from build123d import *

# Parameters (mm, degrees)
F0_W     = 10
F0_H     = 7.475247
F1_DEPTH = 33.528


with BuildPart() as f1:
    # F0 (on Top) → F1 (new body)
    with BuildSketch(Plane.XY):
        with Locations((-52.5, -26.262377)):
            Rectangle(F0_W, F0_H)
        with Locations((52.5, -26.262377)):
            Rectangle(F0_W, F0_H)
        with BuildLine():
            Line((47.5, 30), (-47.5, 30))
            Line((-47.5, 30), (-47.5, -22.524753))
            Line((-47.5, -22.524753), (-47.5, -30))
            Line((-47.5, -30), (-22.5, -30))
            Line((-22.5, -30), (-22.5, 0))
            Line((-22.5, 0), (-22.5, 16.022185))
            ThreePointArc((-22.5, 16.022185), (0, 27.621738), (22.5, 16.022185))
            Line((22.5, 16.022185), (22.5, 0))
            Line((22.5, 0), (22.5, -30))
            Line((22.5, -30), (47.5, -30))
            Line((47.5, -30), (47.5, -22.524753))
            Line((47.5, -22.524753), (47.5, 30))
        make_face()
    extrude(amount=F1_DEPTH)


solid = f1.part
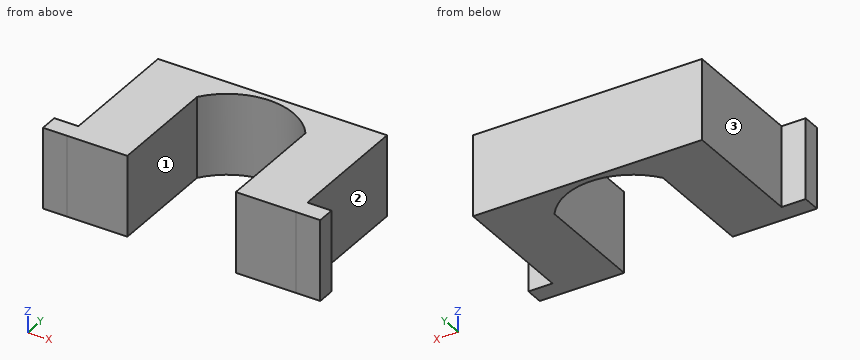
The listing builds one solid part. Answer for the finished solid, in the listing's coordinates (mm). Face numbers are marked on the shaded views. A direction names the side the tool comes from. Coordinates: 2 decimals unless noted, no trailing zeros. Write each loop counter-clockwise with the first axis right and the second up, starting at its lowest first coordinate (ties: lowest second). Pieces come first, ordered by that corner, then holes. Notation, with made-up numbers: (-6, 39.25) - (41, 39.25) arc R33 cw to (41, 73.25) - close; hole circle Ø6 at (83, -22.5). An arc over 180 degrees is marked (long way). Answer as CSV lines item,"result".
1. A tool of negligible diameter and unlimited length cuts with its end or side. For the marked faces 1, 2 and 3, from which of +Z, -Z, +X, -X, +Y, -Y can it reach the whole face along a straight path? Write none if from no direction.
Computed values:
face 1,"+Z, -Z, -Y"
face 2,"+Z, -Z, +X, +Y"
face 3,"+Z, -Z, -X, +Y"
2. Straight lines are drawn through the part: line 1 (X direction, y = 5, z = 17.5); line 2 (Y direction, x = 51.5, z = 24); line 3 (Y direction, x = -16, z = 30). For each, find the intervals that lie inside material, in ascending order. Write a range as [from, to].
Computed values:
line 1,"x = [-47.5, -22.5], [22.5, 47.5]"
line 2,"y = [-30, -22.52]"
line 3,"y = [22.52, 30]"
3. Given P1, Ø1, axis at y = 13.5, z = 26, coming from the -X side; P2, Ø1.5, axis at y = -4.5, z = 13.5, coming from the +X side; P3, Ø8, axis at x = 53.5, z = 9.5, coming from the +Y side, each flat-ended and moving along its own axis, determine where each tip first touches the part or whether it passes through.
Computed values:
P1,"stops at x = -47.5"
P2,"stops at x = 47.5"
P3,"stops at y = -22.52"
4. Find section A-A (y = 0). Give the vertices of the cut face in (x, z), plus the area to 3 significant figures.
Computed values:
outline,"(-47.5, 0) - (-22.5, 0) - (-22.5, 33.53) - (-47.5, 33.53) - close; (22.5, 0) - (47.5, 0) - (47.5, 33.53) - (22.5, 33.53) - close"
area,"1,680 mm²"
5. Find section B-B (z = 17). Give the vertices of the cut face in (x, y), plus the area to 3 significant figures.
Computed values:
outline,"(-57.5, -30) - (-22.5, -30) - (-22.5, 16.02) arc R27.62 cw to (22.5, 16.02) - (22.5, -30) - (57.5, -30) - (57.5, -22.52) - (47.5, -22.52) - (47.5, 30) - (-47.5, 30) - (-47.5, -22.52) - (-57.5, -22.52) - close"
area,"3,410 mm²"
6. Find section C-C (y = 19). Give the vertices of the cut face in (x, z), plus the area to 3 significant figures.
Computed values:
outline,"(-47.5, 0) - (-20.05, 0) - (-20.05, 33.53) - (-47.5, 33.53) - close; (20.05, 0) - (47.5, 0) - (47.5, 33.53) - (20.05, 33.53) - close"
area,"1,840 mm²"
7. Find section D-D (x = -13). Give the vertices of the cut face in (y, z).
Computed values:
outline,"(24.37, 0) - (30, 0) - (30, 33.53) - (24.37, 33.53) - close"
